For this review, take the finished solid that the model builds, in its own axes (mm). Face numbers are marked on the shaded views. A direction names the side the tool comes from. Coordinates: 2 decimals unless noted, no trailing zeros. Write each loop counter-clockwise with the first axis right and the second up, starting at its lowest first coordinate (ties: lowest second). Pieces come first, ordered by that corner, then holes. Notation, with made-up numbers: M 30,-22.5 L 58,-22.5 A20 cw 58,-17.5 Z; hole C 3.5,84.25 d5. An arc over 180 degrees is marked long. One line per question, with ' | ' between items.
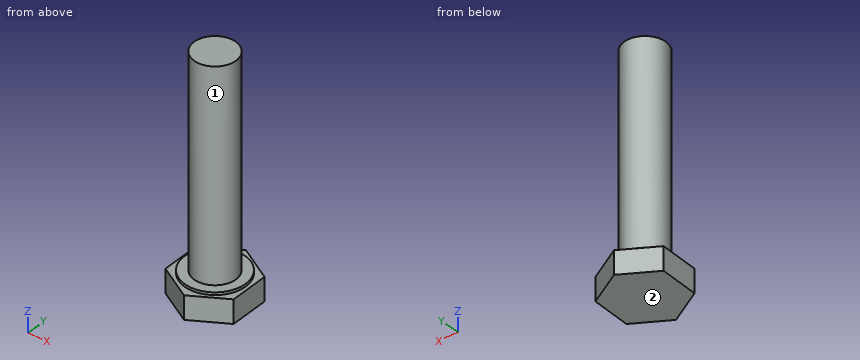
from build123d import *

# Parameters (mm, degrees)
BOSS_EXTRUDE1_DEPTH = 4.5
SKETCH2_R           = 5.85
BOSS_EXTRUDE2_DEPTH = 0.5
SKETCH3_R           = 4
BOSS_EXTRUDE3_DEPTH = 40


with BuildPart() as part:
    # Sketch1 → Boss-Extrude1 (new body)
    with BuildSketch(Plane.XY):
        Polygon((-6.411545587, -3.901975976), (0.173437527, -7.503549344), (6.584983114, -3.601573368), (6.411545587, 3.901975976), (-0.173437527, 7.503549344), (-6.584983114, 3.601573368), align=None)
    extrude(amount=BOSS_EXTRUDE1_DEPTH)

    # Sketch2 → Boss-Extrude2 (add)
    with BuildSketch(Plane.XY.offset(4.5)):
        Circle(SKETCH2_R)
    extrude(amount=BOSS_EXTRUDE2_DEPTH)

    # Sketch3 → Boss-Extrude3 (add)
    with BuildSketch(Plane.XY.offset(5)):
        Circle(SKETCH3_R)
    extrude(amount=BOSS_EXTRUDE3_DEPTH)


solid = part.part
1. Take a section at C-C on z = 30.5. State the section outline as (x, y) points.
Computed values:
outline: C 0,0 d8
2. Machinability: for the marked faces 1 and 2, which of the approach directions +Z, -Z, +X, -X, +Y, -Y give a long, thin tool a straight path to every point of the face, cutting with its end or side? Answer none if there is none.
Computed values:
face 1: +Z | face 2: -Z, +X, -X, +Y, -Y
3. Take a section at B-B on y = -5.25. State the section outline as (x, z) points.
Computed values:
outline: M -3.95,0 L 3.88,0 L 3.88,4.5 L 2.58,4.5 L 2.58,5 L -2.58,5 L -2.58,4.5 L -3.95,4.5 Z
4. Take a section at A-A on x = 4.75. State the section outline as (y, z) points.
Computed values:
outline: M -4.72,0 L 4.81,0 L 4.81,4.5 L 3.41,4.5 L 3.41,5 L -3.41,5 L -3.41,4.5 L -4.72,4.5 Z
5. Clearance check with flat-ended pins moving along their axes: P1, Ø8, axis at y = 2, z = 35.5, coming from the -X side; P2, Ø3, axis at x = 5, z = 20.5, coming from the +Y side; P3, Ø5, axis at y = -4, z = 35, coming from the +X side; P4, Ø5, axis at x = -5, y = -1.5, coming from the +Z side. State where each tip first meets the part, or that it passes through.
Computed values:
P1: stops at x = -4 | P2: stops at y = 1.94 | P3: stops at x = 3.71 | P4: stops at z = 45
6. Take a section at D-D on x = -3. State the section outline as (y, z) points, plus the area to 3 significant figures.
Computed values:
outline: M -5.77,0 L 5.78,0 L 5.78,4.5 L 5.02,4.5 L 5.02,5 L 2.65,5 L 2.65,45 L -2.65,45 L -2.65,5 L -5.02,5 L -5.02,4.5 L -5.77,4.5 Z | area: 269 mm2
7. For line 1 along Z through (x, y) = (-3.25, -5.5); line 2 along Y through (x, z) = (1.75, 28); line 3 along Z through (x, y) = (-4, -0.5), list the stretches that pass through material, from the lowest coordinate up.
Computed values:
line 1: z = 0 to 4.5 | line 2: y = -3.6 to 3.6 | line 3: z = 0 to 5
